```python
from build123d import *

# Parameters (mm, degrees)
SKETCH2_W              = 80
SKETCH2_H              = 60
FLOOR_2_DEPTH          = 2.4
LOWER_WALLS_START      = 2.4
SKETCH3_W              = 80
SKETCH3_H              = 60
SKETCH3_W_2            = 69.2
SKETCH3_H_2            = 49.2
LOWER_WALLS_DEPTH      = 32.3
OUTER_GROOVE_LIP_START = 34.7
SKETCH4_W              = 80
SKETCH4_H              = 60
SKETCH4_W_2            = 77.8
SKETCH4_H_2            = 57.8
OUTER_GROOVE_LIP_DEPTH = 1.3
INNER_GROOVE_LIP_START = 34.7
SKETCH5_W              = 71.4
SKETCH5_H              = 51.4
SKETCH5_W_2            = 69.2
SKETCH5_H_2            = 49.2
INNER_GROOVE_LIP_DEPTH = 1.3
SCREW_BOSS_START       = 2.4
SKETCH6_R              = 4
SKETCH6_R_2            = 1.25
SCREW_BOSS_DEPTH       = 33.8
BOSS_EXTRUDE6_START    = 2.4
SKETCH7_R              = 4
SKETCH7_R_2            = 1.25
BOSS_EXTRUDE6_DEPTH    = 33.8
BOSS_EXTRUDE7_START    = 2.4
SKETCH8_R              = 4
SKETCH8_R_2            = 1.25
BOSS_EXTRUDE7_DEPTH    = 33.8
BOSS_EXTRUDE8_START    = 2.4
SKETCH9_R              = 4
SKETCH9_R_2            = 1.25
BOSS_EXTRUDE8_DEPTH    = 33.8
PCB_POST_START         = 2.4
SKETCH10_R             = 3
SKETCH10_R_2           = 1.4
PCB_POST_DEPTH         = 6
BOSS_EXTRUDE10_START   = 2.4
SKETCH11_R             = 3
SKETCH11_R_2           = 1.4
BOSS_EXTRUDE10_DEPTH   = 6
BOSS_EXTRUDE11_START   = 2.4
SKETCH12_R             = 3
SKETCH12_R_2           = 1.4
BOSS_EXTRUDE11_DEPTH   = 6
BOSS_EXTRUDE12_START   = 2.4
SKETCH13_R             = 3
SKETCH13_R_2           = 1.4
BOSS_EXTRUDE12_DEPTH   = 6


with BuildPart() as part:
    # Sketch2 → Floor 2 (new body)
    with BuildSketch(Plane.XY):
        Rectangle(SKETCH2_W, SKETCH2_H)
    extrude(amount=FLOOR_2_DEPTH)

    # Sketch3 → Lower_walls (add)
    with BuildSketch(Plane.XY.offset(LOWER_WALLS_START)):
        Rectangle(SKETCH3_W, SKETCH3_H)
        Rectangle(SKETCH3_W_2, SKETCH3_H_2, mode=Mode.SUBTRACT)
    extrude(amount=LOWER_WALLS_DEPTH)

    # Sketch4 → Outer_groove_lip (add)
    with BuildSketch(Plane.XY.offset(OUTER_GROOVE_LIP_START)):
        Rectangle(SKETCH4_W, SKETCH4_H)
        Rectangle(SKETCH4_W_2, SKETCH4_H_2, mode=Mode.SUBTRACT)
    extrude(amount=OUTER_GROOVE_LIP_DEPTH)

    # Sketch5 → Inner_groove_lip (add)
    with BuildSketch(Plane.XY.offset(INNER_GROOVE_LIP_START)):
        Rectangle(SKETCH5_W, SKETCH5_H)
        Rectangle(SKETCH5_W_2, SKETCH5_H_2, mode=Mode.SUBTRACT)
    extrude(amount=INNER_GROOVE_LIP_DEPTH)

    # Sketch6 → Screw_boss (add)
    with BuildSketch(Plane.XY.offset(SCREW_BOSS_START)):
        with Locations(Location((-30, -20, 0), (0, 0, 180))):
            Circle(SKETCH6_R)
        with Locations((-30, -20)):
            Circle(SKETCH6_R_2, mode=Mode.SUBTRACT)
    extrude(amount=SCREW_BOSS_DEPTH)

    # Sketch7 → Boss-Extrude6 (add)
    with BuildSketch(Plane.XY.offset(BOSS_EXTRUDE6_START)):
        with Locations(Location((-30, 20, 0), (0, 0, 180))):
            Circle(SKETCH7_R)
        with Locations((-30, 20)):
            Circle(SKETCH7_R_2, mode=Mode.SUBTRACT)
    extrude(amount=BOSS_EXTRUDE6_DEPTH)

    # Sketch8 → Boss-Extrude7 (add)
    with BuildSketch(Plane.XY.offset(BOSS_EXTRUDE7_START)):
        with Locations(Location((30, -20, 0), (0, 0, 180))):
            Circle(SKETCH8_R)
        with Locations((30, -20)):
            Circle(SKETCH8_R_2, mode=Mode.SUBTRACT)
    extrude(amount=BOSS_EXTRUDE7_DEPTH)

    # Sketch9 → Boss-Extrude8 (add)
    with BuildSketch(Plane.XY.offset(BOSS_EXTRUDE8_START)):
        with Locations(Location((30, 20, 0), (0, 0, 180))):
            Circle(SKETCH9_R)
        with Locations((30, 20)):
            Circle(SKETCH9_R_2, mode=Mode.SUBTRACT)
    extrude(amount=BOSS_EXTRUDE8_DEPTH)

    # Sketch10 → PCB_post (add)
    with BuildSketch(Plane.XY.offset(PCB_POST_START)):
        with Locations(Location((-21, -8.5, 0), (0, 0, 180))):
            Circle(SKETCH10_R)
        with Locations((-21, -8.5)):
            Circle(SKETCH10_R_2, mode=Mode.SUBTRACT)
    extrude(amount=PCB_POST_DEPTH)

    # Sketch11 → Boss-Extrude10 (add)
    with BuildSketch(Plane.XY.offset(BOSS_EXTRUDE10_START)):
        with Locations(Location((-21, 8.5, 0), (0, 0, 180))):
            Circle(SKETCH11_R)
        with Locations((-21, 8.5)):
            Circle(SKETCH11_R_2, mode=Mode.SUBTRACT)
    extrude(amount=BOSS_EXTRUDE10_DEPTH)

    # Sketch12 → Boss-Extrude11 (add)
    with BuildSketch(Plane.XY.offset(BOSS_EXTRUDE11_START)):
        with Locations(Location((21, -8.5, 0), (0, 0, 180))):
            Circle(SKETCH12_R)
        with Locations((21, -8.5)):
            Circle(SKETCH12_R_2, mode=Mode.SUBTRACT)
    extrude(amount=BOSS_EXTRUDE11_DEPTH)

    # Sketch13 → Boss-Extrude12 (add)
    with BuildSketch(Plane.XY.offset(BOSS_EXTRUDE12_START)):
        with Locations(Location((21, 8.5, 0), (0, 0, 180))):
            Circle(SKETCH13_R)
        with Locations((21, 8.5)):
            Circle(SKETCH13_R_2, mode=Mode.SUBTRACT)
    extrude(amount=BOSS_EXTRUDE12_DEPTH)


solid = part.part
```
Can you work these out from the model? Positions are in its coordinate system, mm. Coordinates: 2 decimals unless noted, no trailing zeros.
Item 1: Suppose I cut it at A-A (z = 33). State how many separate pieces and enclosed holes the cut face has, then the cut area to 3 significant figures.
Answers below:
separate pieces: 5
enclosed holes: 5
area: 1,580 mm2
Item 2: Please list where these lines run through material, in increasing order: L1, parallel to Y at x = 30, z = 10; L2, parallel to Y at x = -21, z = 6; L3, parallel to Y at x = 19.5, z = 17.
Answers below:
L1: y = -30 to -24.6, -24 to -21.25, -18.75 to -16, 16 to 18.75, 21.25 to 24, 24.6 to 30
L2: y = -30 to -24.6, -11.5 to -9.9, -7.1 to -5.5, 5.5 to 7.1, 9.9 to 11.5, 24.6 to 30
L3: y = -30 to -24.6, 24.6 to 30
Item 3: If we mould it in two halves opening along X, with no side actions, what happens to faces 1 (the face through (-1, 30, 18)), 2 (the face through (30, 20, 2.4))? For each: released by +X, released by -X, zero draft, split by the parting line, or undercut.
Answers below:
face 1: zero draft
face 2: undercut
Item 4: I'm going to push flat-ended pins straight in: pin 1 (2 mm diameter, centred on x = 21.5, y = -9, fed in from +Z); pin 2 (1.2 mm diameter, centred on x = -30, y = 20, fed in from +Z). Where does each tip first touch, or does it pass through?
Answers below:
pin 1: stops at z = 8.4
pin 2: stops at z = 2.4
